Input: part model. Units: mm. Frame: model coordinates. A direction names the side the tool comes from. Give positions to 0.01 mm unless a question says otherwise; leave off trailing zeros. Loops run counter-clockwise (first coordinate to the right, second up) from the corner with the lowest first, then second, coordinate; pieces in that order, holes last. Notation, with made-up numbers: M 59.25,51.5 L 90.25,51.5 A10 ccw 90.25,65.5 Z; hole C 31,58.5 d11. An arc over 180 degrees is marked long. Use CSV: the item, a comma, the result in double quotes. Start each with the question number.
Q1. Section A-A, the plane y = 2.6. Output: boundary loops of the cut face in (x, z), plus the area to 3 significant figures.
Q2. Section D-D, the plane z = -11.25. Output: boundary loops of the cut face in (x, y), plus the area to 3 significant figures.
Q3. Section B-B, the plane z = -3.5. Output: boundary loops of the cut face in (x, y).
Q4. Reachability of faces 1 (the flat face through (-30.239, 4, -1)), 2 (the cylindrical face through (-12.038, 0.986, -7.543)), 3 (the flat face through (-7, 3, 11.385)) from +Z, -Z, +X, -X, +Y, -Y: full face, straight path, thin tool, end or side. Return the list, or none.
Q5. Pin query (flat end, axial travel): pin 1 (13 mm diameter, centred on x = -20.36, z = -2.06, fed in from -Y); pin 2 (2 mm diameter, centred on x = 10.5, z = 4.5, fed in from +Y); pin 3 (12 mm diameter, centred on x = -22.5, z = -10, fed in from +Y). Return the tip coordinate at first contact, or that it passes through.
Q6. Section C-C, the plane x = 11. Output: boundary loops of the cut face in (y, z).
Q7. Pull-direction query (Z, two-part tool) for faces 4 (the flat face through (-7, 3, -14.115)), 5 (the cylindrical face through (-12.308, 1.014, -3.12)), 6 (the flat face through (18.261, 3, -1)); classes: released by +Z, released by -Z, zero draft, split by the parting line, or undercut.
Q8. Material intervals for line 1 along X through (y, z) = (0.4, -2); line 2 along Z through (x, y) = (-3, 1.95); line 3 along X through (y, z) = (2.1, -3.5), sorted ascending.
from build123d import *

# Parameters (mm, degrees)
SKETCH1_W               = 50.5
SKETCH1_H               = 25.5
BOSS_EXTRUDE1_DEPTH     = 2
MOVE_FACE1_BY           = 5
CUT_EXTRUDE1_DEPTH      = 12
CUT_EXTRUDE1_DEPTH_BACK = 0.0001
SKETCH2_W               = 46.5
SKETCH2_H               = 21.5
SKETCH3_R               = 8.125
CUT_EXTRUDE2_DEPTH      = 10.0001
SKETCH4_W               = 11
SKETCH4_H               = 5
CUT_EXTRUDE3_DEPTH      = 10.0001
FILLET1_R               = 1.5
SKETCH5_W               = 10
SKETCH5_H               = 2
CUT_EXTRUDE4_DEPTH      = 10.0001
FILLET2_R               = 1
MOVE_START              = 6
MOVE_FACE2_OUTLINE_W    = 50.5
MOVE_FACE2_OUTLINE_H    = 25.5
MOVE_FACE2_OUTLINE_W_2  = 46.5
MOVE_FACE2_OUTLINE_H_2  = 21.5
MOVE_FACE2_DEPTH        = 1


# Read off the part's stored shape, not the designer's step: Move Face2
with BuildPart() as part:
    # Sketch1 → Boss-Extrude1 (new body)
    with BuildSketch(Plane(origin=(0, 0, 0), x_dir=(1, 0, 0), z_dir=(0, 1, 0))):
        with Locations((-6.98861547, 1.365023474)):
            Rectangle(SKETCH1_W, SKETCH1_H)
    extrude(amount=BOSS_EXTRUDE1_DEPTH)

    # Move Face1: a face moved outward by 5.0
    extrude(part.faces().sort_by_distance((-6.98861547, 2, -1.365023474))[0], amount=MOVE_FACE1_BY, dir=(0, 1, 0))

    # Sketch2 → Cut-Extrude1 (cut, two sides: drawn at the far end of the back side and taken through both)
    with BuildSketch(Plane(origin=(0, 2, 0), x_dir=(1, 0, 0), z_dir=(0, 1, 0)).offset(-CUT_EXTRUDE1_DEPTH_BACK)):
        with Locations((-6.98861547, 1.365023474)):
            Rectangle(SKETCH2_W, SKETCH2_H)
    extrude(amount=CUT_EXTRUDE1_DEPTH + CUT_EXTRUDE1_DEPTH_BACK, mode=Mode.SUBTRACT)

    # Sketch3 → Cut-Extrude2 (cut)
    with BuildSketch(Plane(origin=(0, 1.9999, 0), x_dir=(1, 0, 0), z_dir=(0, 1, 0))):
        with Locations(Location((-20.36361547, 2.06192688, 0), (0, 0, 270))):
            Circle(SKETCH3_R)
        with Locations(Location((6.38638453, 1.683174436, 0), (0, 0, 270))):
            Circle(SKETCH3_R)
    extrude(amount=-CUT_EXTRUDE2_DEPTH, mode=Mode.SUBTRACT)

    # Sketch4 → Cut-Extrude3 (cut)
    with BuildSketch(Plane(origin=(0, 1.9999, 0), x_dir=(1, 0, 0), z_dir=(0, 1, 0))):
        with Locations((-6.98861547, 9.615023474)):
            Rectangle(SKETCH4_W, SKETCH4_H)
    extrude(amount=-CUT_EXTRUDE3_DEPTH, mode=Mode.SUBTRACT)

    # Fillet1
    fillet1_edges = [part.edges().sort_by_distance(p)[0] for p in [
        (-12.48861547, 0.99995, -7.115023474),
        (-12.48861547, 0.99995, -12.115023474),
        (-1.48861547, 0.99995, -12.115023474),
        (-1.48861547, 0.99995, -7.115023474),
    ]]
    fillet(fillet1_edges, radius=FILLET1_R)

    # Sketch5 → Cut-Extrude4 (cut)
    with BuildSketch(Plane(origin=(0, 1.9999, 0), x_dir=(1, 0, 0), z_dir=(0, 1, 0))):
        with Locations((-6.98861547, -8.384976526)):
            Rectangle(SKETCH5_W, SKETCH5_H)
    extrude(amount=-CUT_EXTRUDE4_DEPTH, mode=Mode.SUBTRACT)

    # Fillet2
    fillet2_edges = [part.edges().sort_by_distance(p)[0] for p in [
        (-1.98861547, 0.99995, 9.384976526),
        (-1.98861547, 0.99995, 7.384976526),
        (-11.98861547, 0.99995, 7.384976526),
        (-11.98861547, 0.99995, 9.384976526),
    ]]
    fillet(fillet2_edges, radius=FILLET2_R - 0.0001)  # a hair under: the kernel refuses the full size

    # Move Face2 outline → Move Face2 (cut)
    with BuildSketch(Plane(origin=(0, 0, 0), x_dir=(1, 0, 0), z_dir=(0, 1, 0)).offset(MOVE_START)):
        with Locations((-6.98861547, 1.365023474)):
            Rectangle(MOVE_FACE2_OUTLINE_W, MOVE_FACE2_OUTLINE_H)
        with Locations((-6.98861547, 1.365023474)):
            Rectangle(MOVE_FACE2_OUTLINE_W_2, MOVE_FACE2_OUTLINE_H_2, mode=Mode.SUBTRACT)
    extrude(amount=MOVE_FACE2_DEPTH, mode=Mode.SUBTRACT)


solid = part.part
A:
1,outline,"M -32.24,-14.12 L 18.26,-14.12 L 18.26,11.38 L -32.24,11.38 Z; hole M -30.24,-12.12 L 16.26,-12.12 L 16.26,9.38 L -30.24,9.38 Z"
1,area,"288 mm^2"
2,outline,"M -32.24,0 L -12.35,0 L -12.35,2 L -30.24,2 L -30.24,6 L -32.24,6 Z; M -1.63,0 L 18.26,0 L 18.26,6 L 16.26,6 L 16.26,2 L -1.63,2 Z"
2,area,"95.6 mm^2"
3,outline,"M -32.24,0 L -28.36,0 L -28.36,2 L -30.24,2 L -30.24,6 L -32.24,6 Z; M -12.37,0 L -1.53,0 L -1.53,2 L -12.37,2 Z; M 14.31,0 L 18.26,0 L 18.26,6 L 16.26,6 L 16.26,2 L 14.31,2 Z"
4,face 1,"+Y"
4,face 2,"+Y, -Y"
4,face 3,"+Z, +X, -X, +Y, -Y"
5,pin 1,"through"
5,pin 2,"y = 2"
5,pin 3,"y = 6"
6,outline,"M 0,-14.12 L 6,-14.12 L 6,-12.12 L 2,-12.12 L 2,-8.37 L 0,-8.37 Z; M 0,5 L 2,5 L 2,9.38 L 6,9.38 L 6,11.38 L 0,11.38 Z"
7,face 4,"released by -Z"
7,face 5,"undercut"
7,face 6,"zero draft"
8,line 1,"-32.24 to -28.49, -12.24 to -1.73, 14.51 to 18.26"
8,line 2,"-14.12 to -12.12, -7.12 to 7.38, 9.38 to 11.38"
8,line 3,"-32.24 to -30.24, 16.26 to 18.26"
